```python
from build123d import *

# Parameters (mm, degrees)
SKETCH1_R               = 10
BOSS_EXTRUDE1_DEPTH     = 7.5
CUT_EXTRUDE1_DEPTH      = 8.5
SKETCH3_R               = 4
BOSS_EXTRUDE2_DEPTH     = 1
SKETCH3_3_W             = 2
SKETCH3_3_H             = 1.333333333
CUT_EXTRUDE2_DEPTH      = 2
CUT_EXTRUDE2_DEPTH_BACK = 17
CIRPATTERN2_COUNT       = 8


with BuildPart() as part:
    # Sketch1 → Boss-Extrude1 (new body, symmetric)
    with BuildSketch(Plane.XY):
        Circle(SKETCH1_R)
    extrude(amount=BOSS_EXTRUDE1_DEPTH, both=True)

    # Sketch2 → Cut-Extrude1 (cut, symmetric)
    with BuildSketch(Plane.XY):
        with BuildLine():
            ThreePointArc((0.919743931, 5.422552084), (0, 5.5), (-0.919743931, 5.422552084))
            ThreePointArc((-0.919743931, 5.422552084), (-1.482705591, 7.626183267), (-2.398327114, 9.708142307))
            ThreePointArc((-2.398327114, 9.708142307), (0, 10), (2.398327114, 9.708142307))
            ThreePointArc((2.398327114, 9.708142307), (1.482705591, 7.626183267), (0.919743931, 5.422552084))
        make_face()
    cut_extrude1 = extrude(amount=CUT_EXTRUDE1_DEPTH, both=True, mode=Mode.SUBTRACT)

    # Sketch3 → Boss-Extrude2 (add, symmetric)
    with BuildSketch(Plane.XY.offset(7.5)):
        Circle(SKETCH3_R)
        with BuildLine():
            Line((-1, 2.828427125), (-1, 3.495093791))
            Line((-1, 3.495093791), (1, 3.495093791))
            Line((1, 3.495093791), (1, 2.828427125))
            ThreePointArc((1, 2.828427125), (0, -3), (-1, 2.828427125))
        make_face(mode=Mode.SUBTRACT)
    boss_extrude2 = extrude(amount=BOSS_EXTRUDE2_DEPTH, both=True)

    # Mirror1: Boss-Extrude2 across plane
    add(boss_extrude2.mirror(Plane.XY))

    # Sketch3<3> → Cut-Extrude2 (cut, two sides)
    with BuildSketch(Plane.XY.offset(7.5)) as cut_extrude2_sk:
        with BuildLine():
            Line((-1, 2.161760458), (-1, 2.828427125))
            ThreePointArc((-1, 2.828427125), (0, -3), (1, 2.828427125))
            Line((1, 2.828427125), (1, 2.161760458))
            Line((1, 2.161760458), (-1, 2.161760458))
        make_face()
        with Locations((0, 2.828427125)):
            Rectangle(SKETCH3_3_W, SKETCH3_3_H)
    extrude(amount=CUT_EXTRUDE2_DEPTH, mode=Mode.SUBTRACT)
    extrude(cut_extrude2_sk.sketch, amount=-CUT_EXTRUDE2_DEPTH_BACK, mode=Mode.SUBTRACT)

    # CirPattern2: Cut-Extrude1 ×8 about axis
    cirpattern2_axis = Axis((0, 0, 0), (0, 0, 1))
    for i in range(1, CIRPATTERN2_COUNT):
        add(cut_extrude1.rotate(cirpattern2_axis, i * 360 / CIRPATTERN2_COUNT), mode=Mode.SUBTRACT)


solid = part.part
```
Part model, mm, in its own coordinate system. A direction names the side the tool comes from. Round coordinates to 2 decimals unless told otherwise and drop trailing zeros. Loops run counter-clockwise (first coordinate to the right, second up) from the corner with the lowest first, then second, coordinate; pieces in that order, holes last.
Item 1: Drill centre lines: line 1 (X direction, y = 0, z = -8.1); line 2 (Y direction, x = 4, z = -6.5); line 3 (Y direction, x = 0, z = -8.15). Where is each one in solid material? Low to high.
Item 2: Cut at C-C, the plane y = -7. Give the cut face in (x, z), then the cut area to 3 significant figures.
Item 3: Drop flat-ended pins along their axis: P1, Ø0.6, axis at x = 0, z = 0, coming from the -Y side; P2, Ø1.5, axis at x = -6.5, z = -6.5, coming from the +Y side; P3, Ø0.5, axis at x = 0.5, z = 8, coming from the -Y side. Give the stop position or say it passes through.
Item 4: 3-axis set-ups, long thin cutter, end or side, ignore diameter. For faces 1 (the face through (4.36, -6.47, 0.11)), 2 (the face through (-7.656, 1.493, 0.105)), 3 (the face through (1.493, 7.656, 0.105)), 4 (the face through (7.596, 1.472, 0.105)): which of +Z, -Z, +X, -X, +Y, -Y reach the whole face in a straight line?
Item 5: Cut at D-D, the plane x = -2. Give the cut face in (y, z), then the cut area to 3 significant figures.
Item 6: Cut at A-A, the plane x = 0. Give the cut face in (y, z), then the cut area to 3 significant figures.
Item 7: Mould opens along X. For faces 5 (the face through (-5.5, 0, 0.1)), 6 (the face through (3.807, -9.247, 0.105)), 7 (the face through (6.47, 4.36, 0.11)) say: +X half, -X half, draft (parallel to the pull), parting line (faces both ways), or undercut.
Item 8: Cut at B-B, the plane y = 0. Give the cut face in (x, z), then the cut area to 3 significant figures.
A:
1. line 1: x = -4 to -3, 3 to 4
1. line 2: y = -9.17 to -5.78, -3.77 to 3.77, 5.78 to 9.17
1. line 3: y = -4 to -3, 3.5 to 4
2. outline: (-4.6, -7.5) - (-1.28, -7.5) - (-1.28, 7.5) - (-4.6, 7.5) - close; (1.28, -7.5) - (4.6, -7.5) - (4.6, 7.5) - (1.28, 7.5) - close
2. area: 99.5 mm2
3. P1: stops at y = -5.5
3. P2: stops at y = 4.71
3. P3: stops at y = -3.99
4. face 1: +Z, -Z
4. face 2: +Z, -Z, -X
4. face 3: +Z, -Z, +Y
4. face 4: +Z, -Z, +X
5. outline: (-8.91, -7.5) - (-3.46, -7.5) - (-3.46, -8.5) - (-2.24, -8.5) - (-2.24, 8.5) - (-3.46, 8.5) - (-3.46, 7.5) - (-8.91, 7.5) - close; (2.24, -8.5) - (3.46, -8.5) - (3.46, -7.5) - (8.91, -7.5) - (8.91, 7.5) - (3.46, 7.5) - (3.46, 8.5) - (2.24, 8.5) - close
5. area: 205 mm2
6. outline: (-5.5, -7.5) - (-4, -7.5) - (-4, -8.5) - (-3, -8.5) - (-3, 8.5) - (-4, 8.5) - (-4, 7.5) - (-5.5, 7.5) - close; (3.5, -8.5) - (4, -8.5) - (4, -7.5) - (5.5, -7.5) - (5.5, 7.5) - (4, 7.5) - (4, 8.5) - (3.5, 8.5) - close
6. area: 70.6 mm2
7. face 5: -X half
7. face 6: +X half
7. face 7: undercut
8. outline: (-5.5, -7.5) - (-4, -7.5) - (-4, -8.5) - (-3, -8.5) - (-3, 8.5) - (-4, 8.5) - (-4, 7.5) - (-5.5, 7.5) - close; (3, -8.5) - (4, -8.5) - (4, -7.5) - (5.5, -7.5) - (5.5, 7.5) - (4, 7.5) - (4, 8.5) - (3, 8.5) - close
8. area: 79.0 mm2
